from build123d import *

# Parameters (mm, degrees)
SKETCH_1_W          = 11.999999915
SKETCH_1_H          = 11.994665989
SKETCH_1_W_2        = 11.999999916
SKETCH_1_H_2        = 12.000914401
SKETCH_1_W_3        = 68.2
SKETCH_1_H_3        = 30.6
EXTRUDE_1_DEPTH     = 2.4
CUT_EXTRUDE_1_DEPTH = 1.3
FILLET_1_R          = 4


with BuildPart() as part:
    # 草图1 → 凸台-拉伸1 (new body)
    with BuildSketch(Plane(origin=(0, 0, 0), x_dir=(1, 0, 0), z_dir=(0, 1, 0))):
        with BuildLine():
            Line((4.2, -0.1), (88.17478029, -0.1))
            ThreePointArc((88.17478029, -0.1), (91.073918092, -1.300862197), (92.27478029, -4.2))
            Line((92.27478029, -4.2), (92.27478029, -53.174709169))
            ThreePointArc((92.27478029, -53.174709169), (91.073918092, -56.073846972), (88.17478029, -57.274709169))
            Line((88.17478029, -57.274709169), (4.2, -57.274709169))
            ThreePointArc((4.2, -57.274709169), (1.300862197, -56.073846972), (0.1, -53.174709169))
            Line((0.1, -53.174709169), (0.1, -4.2))
            ThreePointArc((0.1, -4.2), (1.300862197, -1.300862197), (4.2, -0.1))
        make_face()
        with Locations((41.319380239, -48.050393701)):
            Rectangle(SKETCH_1_W, SKETCH_1_H, mode=Mode.SUBTRACT)
        with Locations((58.845415291, -48.050393701)):
            Rectangle(SKETCH_1_W, SKETCH_1_H, mode=Mode.SUBTRACT)
        with Locations((76.371450343, -48.047269495)):
            Rectangle(SKETCH_1_W_2, SKETCH_1_H_2, mode=Mode.SUBTRACT)
        with Locations((48.452479045, -21.09040811)):
            Rectangle(SKETCH_1_W_3, SKETCH_1_H_3, mode=Mode.SUBTRACT)
    extrude(amount=EXTRUDE_1_DEPTH)

    # 草图2 → 切除-拉伸1 (cut)
    with BuildSketch(Plane.XZ):
        with BuildLine():
            Line((88.152479045, 39.536375413), (4.206301753, 39.536375413))
            ThreePointArc((4.206301753, 39.536375413), (2.509245478, 38.833431688), (1.806301753, 37.136375413))
            Line((1.806301753, 37.136375413), (1.806301753, 4.190299721))
            ThreePointArc((1.806301753, 4.190299721), (2.509245478, 2.493243446), (4.206301753, 1.790299721))
            Line((4.206301753, 1.790299721), (88.152479045, 1.790299721))
            ThreePointArc((88.152479045, 1.790299721), (89.84953532, 2.493243446), (90.552479045, 4.190299721))
            Line((90.552479045, 4.190299721), (90.552479045, 37.136375413))
            ThreePointArc((90.552479045, 37.136375413), (89.84953532, 38.833431688), (88.152479045, 39.536375413))
        make_face()
    extrude(amount=-CUT_EXTRUDE_1_DEPTH, mode=Mode.SUBTRACT)

    # 圆角1
    fillet_1_edges = [part.edges().sort_by_distance(p)[0] for p in [
        (70.371450385, 1.2, 42.046812294),
        (70.371450385, 1.2, 54.047726695),
        (82.371450301, 1.2, 54.047726695),
        (82.371450301, 1.2, 42.046812294),
        (52.845415333, 1.2, 42.053060706),
        (52.845415333, 1.2, 54.047726695),
        (64.845415248, 1.2, 54.047726695),
        (64.845415248, 1.2, 42.053060706),
        (35.319380281, 1.2, 42.053060706),
        (35.319380281, 1.2, 54.047726695),
        (47.319380196, 1.2, 54.047726695),
        (47.319380196, 1.2, 42.053060706),
    ]]
    fillet(fillet_1_edges, radius=FILLET_1_R)


solid = part.part
Model file for the job. Use its own axes, mm. A direction names the side the tool comes from. Give positions to 0.01 mm unless a question says otherwise; leave off trailing zeros. Loops run counter-clockwise (first coordinate to the right, second up) from the corner with the lowest first, then second, coordinate; pieces in that order, holes last.
Item 1: Mould opens along X. For faces 4 (the face through (47.319, 1, 48)), 5 (the face through (91.11, 1.18, 56.04)), 6 (the face through (47, 2.4, 41)) say: +X half, -X half, draft (parallel to the pull), parting line (faces both ways), or undercut.
Check values:
face 4: undercut
face 5: +X half
face 6: draft
Item 2: Slice it at B-B (z = 14). Write the cut outline in (x, y).
Check values:
outline: (0.1, 0) - (1.81, 0) - (1.81, 1.3) - (14.35, 1.3) - (14.35, 2.4) - (0.1, 2.4) - close; (82.55, 1.3) - (90.55, 1.3) - (90.55, 0) - (92.27, 0) - (92.27, 2.4) - (82.55, 2.4) - close
Item 3: Slice it at D-D (y = 1.85). Give the number of separate pieces and of enclosed holes in the cut face, plus the area to 3 significant figures.
Check values:
separate pieces: 1
enclosed holes: 4
area: 2,780 mm2
Item 4: Slice it at C-C (x = 76.5). Write the cut outline in (y, z).
Check values:
outline: (0, 0.1) - (2.4, 0.1) - (2.4, 5.79) - (1.3, 5.79) - (1.3, 1.79) - (0, 1.79) - close; (0, 39.54) - (1.3, 39.54) - (1.3, 36.39) - (2.4, 36.39) - (2.4, 42.05) - (0, 42.05) - close; (0, 54.05) - (2.4, 54.05) - (2.4, 57.27) - (0, 57.27) - close
Item 5: Slice it at A-A (x = 27.5). Write the cut outline in (y, z).
Check values:
outline: (0, 0.1) - (2.4, 0.1) - (2.4, 5.79) - (1.3, 5.79) - (1.3, 1.79) - (0, 1.79) - close; (0, 39.54) - (1.3, 39.54) - (1.3, 36.39) - (2.4, 36.39) - (2.4, 57.27) - (0, 57.27) - close
Item 6: Which spindle directions (+Z, -Z, +X, -X, +Y, -Y) get a long thin tool onto all of the face, cutting with end or side? Do faces 1 (the face through (2.528, 0.641, 38.852)), 2 (the face through (53.986, 1.217, 52.845)), 3 (the face through (46, 1, 0.1)). Say none if no direction does.
Check values:
face 1: -Y
face 2: +Y, -Y
face 3: -Z, +X, -X, +Y, -Y
Item 7: Drill centre lines: line 1 along Z through (x, y) = (61, 1.8); line 2 along Z through (x, y) = (15, 0.6); line 3 along X through (y, z) = (0.9, 24). Where is each one in solid material? Low to high.
Check values:
line 1: z = 0.1 to 5.79, 36.39 to 42.06, 54.04 to 57.27
line 2: z = 0.1 to 1.79, 39.54 to 57.27
line 3: x = 0.1 to 1.81, 90.55 to 92.27
